Geometry: final body of the model. Coordinates: model frame, mm. A direction names the side the tool comes from. Round coordinates to 2 decimals unless told otherwise and drop trailing zeros. Loops run counter-clockwise (first coordinate to the right, second up) from the corner with the lowest first, then second, coordinate; pieces in that order, holes last. Notation, with made-up numbers: (-31.75, 27) - (4.25, 27) arc R16 ccw to (4.25, 47) - close; hole circle Ø7 at (-15.75, 3.5). An arc over 180 degrees is marked (long way). Answer in a Markdown table with one row per item. Add a question column.
from build123d import *

# Parameters (mm, degrees)
F1_DEPTH  = 12.7
F2_R      = 12.3782206299
F3_DEPTH  = 25.4
F4_W      = 43.5863994062
F4_H      = 31.6992001608
F5_DEPTH  = 7.62
F6_W      = 17.6784005016
F6_H      = 13.8683998957
F7_DEPTH  = 12.7
F8_W      = 17.6784005016
F8_H      = 17.8308002651
F9_DEPTH  = 25.4
F11_DEPTH = 44.45


with BuildPart() as f1:
    # F0 (on Top) → F1 (new body)
    with BuildSketch(Plane.XY):
        Polygon((-66.4464011788, -18.1356016546), (-18.1801488484, -40.3860025108), (18.592800945, -40.3860025108), (66.4464011788, -18.1356016546), (66.4464011788, 17.8308002651), (-66.4464011788, 17.8308002651), align=None)
    extrude(amount=F1_DEPTH)

    # F2 (on face) → F3 (cut)
    with BuildSketch(Plane.XY.offset(12.7)):
        with Locations((50.2920001745, 0)):
            Circle(F2_R)
        with Locations((-50.2920001745, 0)):
            Circle(F2_R)
    extrude(amount=-F3_DEPTH, mode=Mode.SUBTRACT)

    # F4 (on face) → F5 (join)
    with BuildSketch(Plane.XY.offset(12.7)):
        with Locations((4.1147992015, 1.9812001847)):
            Rectangle(F4_W, F4_H)
    extrude(amount=F5_DEPTH)

    # F6 (on face) → F7 (join)
    with BuildSketch(Plane.XY.offset(20.32)):
        with Locations((-8.8392002508, -6.9341999479)):
            Rectangle(F6_W, F6_H)
    extrude(amount=F7_DEPTH)

    # F8 (on face) → F9 (join)
    with BuildSketch(Plane.XY.offset(20.32)):
        with Locations((-8.8392002508, 8.9154001325)):
            Rectangle(F8_W, F8_H)
    extrude(amount=F9_DEPTH)

    # F10 (on face) → F11 (join)
    with BuildSketch(Plane.YZ):
        Polygon((-1.0628e-06, 45.5676019192), (0, 39.37), (17.8308002651, 39.37), (17.8308002651, 45.72), align=None)
    extrude(amount=F11_DEPTH)


solid = f1.part
1) Section D-D, the plane y = -25. Return the cut outline in (x, z), and give its area (3 significant figures).
2) Material intervals for line 1 along Z through (x, y) = (24, 1); line 2 along Z through (x, y) = (-25, -7); line 3 along X through (y, z) = (14.5, 15.5), sorted ascending. Write a range as from..to.
3) Contact query for flat-ended pins moving along their axis: pin 1 Ø5 at (x, z) = (24.5, 42.5) entering from -Y; pin 2 Ø4 at (y, z) = (9.5, 15) entering from +X; pin 3 Ø22.5 at (x, y) = (50.292, 0) entering from +Z. Output: stop coordinate, or through.
4) Reachability of faces 1 (the flat face through (0, 2, 28)), 2 (the flat face through (-17.678, 2, 25)), 3 (the flat face through (-1, -13.868, 20)), 4 (the flat face through (0, -40.386, 6)) from +Z, -Z, +X, -X, +Y, -Y: full face, straight path, thin tool, end or side. Return the list, or none.
5) Section B-B, the plane x = -54.5. Return the cut outline in (y, z).
6) Pull-direction query (Z, two-part tool) for faces 5 (the flat face through (25.908, 2, 16)), 6 (the flat face through (-9, -7, 33.02)), 7 (the flat face through (66.446, 0, 6)), 8 (the flat face through (-1, -11, 0)); classes: pulls with the +Z half, pulls with the -Z half, needs draft (parallel to the pull), parting line crosses it, or undercut.
7) Section A-A, the plane x = -8. Return the cut outline in (y, z).
8) Section C-C, the plane z = 15.5. Return the cut outline in (x, y), and give its area (3 significant figures).
Evaluation:
| question | item | result |
|---|---|---|
| 1 | outline | (-51.56, 0) - (51.68, 0) - (51.68, 12.7) - (-51.56, 12.7) - close |
| 1 | area | 1,310 mm² |
| 2 | line 1 | z = 0..20.32, 39.37..45.58 |
| 2 | line 2 | z = 0..12.7 |
| 2 | line 3 | x = -17.68..25.91 |
| 3 | pin 1 | stops at y = 0 |
| 3 | pin 2 | stops at x = 25.91 |
| 3 | pin 3 | stops at z = 45.65 |
| 4 | face 1 | +X, +Y, -Y |
| 4 | face 2 | +Z, -X, +Y, -Y |
| 4 | face 3 | +Z, +X, -X, -Y |
| 4 | face 4 | +Z, -Z, +X, -X, -Y |
| 5 | outline | (-23.64, 0) - (-11.64, 0) - (-11.64, 12.7) - (-23.64, 12.7) - close; (11.64, 0) - (17.83, 0) - (17.83, 12.7) - (11.64, 12.7) - close |
| 6 | face 5 | undercut |
| 6 | face 6 | pulls with the +Z half |
| 6 | face 7 | needs draft |
| 6 | face 8 | pulls with the -Z half |
| 7 | outline | (-40.39, 0) - (17.83, 0) - (17.83, 45.72) - (0, 45.72) - (0, 33.02) - (-13.87, 33.02) - (-13.87, 12.7) - (-40.39, 12.7) - close |
| 8 | outline | (-17.68, -13.87) - (25.91, -13.87) - (25.91, 17.83) - (-17.68, 17.83) - close |
| 8 | area | 1,380 mm² |
